Part model, mm, in its own coordinate system. Face numbers are marked on the shaded views. A direction names the side the tool comes from. Coordinates: 2 decimals unless noted, no trailing zeros. Loops run counter-clockwise (first coordinate to the right, second up) from the corner with the lowest first, then second, coordinate; pieces in that order, holes last. Notation, with made-up numbers: (52, 60.5) - (81, 60.5) arc R8 cw to (81, 70.5) - close; hole circle Ø9 at (31, -17). An arc over 180 degrees is marked (long way). One line per question, with ' | ' between items. Start each with the question number.
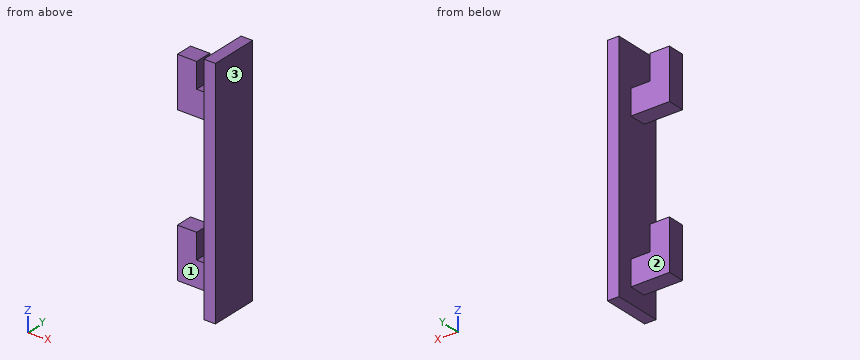
from build123d import *

# Parameters (mm, degrees)
PAD_DEPTH         = 4.4
SKETCH001_W       = 3
SKETCH001_H       = 61
PAD001_DEPTH      = 4
PAD001_DEPTH_BACK = 8.4


with BuildPart() as part:
    # Sketch → Pad (new body)
    with BuildSketch(Plane.XZ):
        Polygon((-3, -30.5), (-3, -26.5), (-13, -26.5), (-13, -13.5), (-8, -13.5), (-8, -20), (-3, -20), (-3, 13.5), (-13, 13.5), (-13, 26.5), (-8, 26.5), (-8, 20), (-3, 20), (-3, 30.5), (0, 30.5), (0, -30.5), align=None)
    extrude(amount=PAD_DEPTH)

    # Sketch001 (on Face18 of Pad) → Pad001 (join, two sides)
    with BuildSketch(Plane.XZ.offset(4.4)) as pad001_sk:
        with Locations((-1.5, 0)):
            Rectangle(SKETCH001_W, SKETCH001_H)
    extrude(amount=PAD001_DEPTH)
    extrude(pad001_sk.sketch, amount=-PAD001_DEPTH_BACK)


solid = part.part
1) Band-saw the part on B-B on y = -2.25. List the corners of the cut face in (x, z).
2) Tool access for the marked faces 1, 2 and 3: list every direction of +Z, -Z, +X, -X, +Y, -Y with a clear straight run to the whole face (end or side of a thin tool).
3) Band-saw the part on D-D on x = -4.5. List the corners of the cut face in (y, z), then the cut area to 3 significant figures.
4) Band-saw the part on C-C on z = 15.5. List the corners of the cut face in (x, y).
5) Pin check, flat tips, straight feed: pin 1 Ø2 at (y, z) = (1, -3.5) entering from -X; pin 2 Ø5 at (x, z) = (-10, 22) entering from +Y; pin 3 Ø2 at (x, y) = (-8.5, -3) entering from -Z. Stop position of each tip, or through.
6) Band-saw the part on A-A on x = -9.25. List the corners of the cut face in (y, z).
7) Wall check: line 1 along Z through (x, y) = (-3.5, -4.25); line 2 along X through (y, z) = (-3, 11); line 3 along Z through (x, y) = (-10, -4). Give the ranges that are in metal, low to high. Write a range as [from, to].
Values found:
1) outline: (-13, -26.5) - (-3, -26.5) - (-3, -30.5) - (0, -30.5) - (0, 30.5) - (-3, 30.5) - (-3, 20) - (-8, 20) - (-8, 26.5) - (-13, 26.5) - (-13, 13.5) - (-3, 13.5) - (-3, -20) - (-8, -20) - (-8, -13.5) - (-13, -13.5) - close
2) face 1: +Z, -Z, -X, -Y | face 2: +Z, -Z, -X, +Y | face 3: +Z, -Z, +X, +Y, -Y
3) outline: (-4.4, -26.5) - (0, -26.5) - (0, -20) - (-4.4, -20) - close; (-4.4, 13.5) - (0, 13.5) - (0, 20) - (-4.4, 20) - close | area: 57.2 mm²
4) outline: (-13, -4.4) - (-3, -4.4) - (-3, -8.4) - (0, -8.4) - (0, 4) - (-3, 4) - (-3, 0) - (-13, 0) - close
5) pin 1: x = -3 | pin 2: y = 0 | pin 3: z = -26.5
6) outline: (-4.4, -26.5) - (0, -26.5) - (0, -13.5) - (-4.4, -13.5) - close; (-4.4, 13.5) - (0, 13.5) - (0, 26.5) - (-4.4, 26.5) - close
7) line 1: [-26.5, -20], [13.5, 20] | line 2: [-3, 0] | line 3: [-26.5, -13.5], [13.5, 26.5]
